from build123d import *

# Parameters (mm, degrees)
SKETCH_1_W                  = 84
SKETCH_1_H                  = 80
SKETCH_1_R                  = 14
EXTRUDE_1_DEPTH             = 5
EXTRUDE_2_DEPTH             = 22
CUT_EXTRUDE_3_REACH         = 79
HOLE_START                  = -42
HOLE_WIZARD_2_OUTLINE_R     = 1.7
HOLE_WIZARD_2_DEPTH         = 11
HOLE_WIZARD_2_2_OUTLINE_R   = 3
HOLE_WIZARD_2_2_OUTLINE_R_2 = 1.7
HOLE_WIZARD_2_2_DEPTH       = 3.4
HOLE_WIZARD_M4_2_D          = 3.3
SKETCH_14_R                 = 38
SKETCH_14_R_2               = 31.1
CUT_EXTRUDE_4_DEPTH         = 4
HOLE_WIZARD_3_D             = 3.2
HOLE_WIZARD_3_CBORE_D       = 6
HOLE_WIZARD_3_CBORE_DEPTH   = 3.4
CHAMFER_1_SIZE              = 23


# Read off the part's stored shape, not the designer's step: 打孔尺寸(%根据)内六角圆柱头螺钉的类型2
with BuildPart() as part:
    # 草图1 → 凸台-拉伸1 (new, symmetric)
    with BuildSketch(Plane.XY):
        Rectangle(SKETCH_1_W, SKETCH_1_H)
        Circle(SKETCH_1_R, mode=Mode.SUBTRACT)
    extrude(amount=EXTRUDE_1_DEPTH, both=True)

    # 草图6 → 凸台-拉伸2 (add)
    with BuildSketch(Plane.ZY.offset(42)):
        Polygon((-5, -14.766158372), (-5, -40), (-30, -40), (-33.816179908, -20.367456331), align=None)
    extrude_2 = extrude(amount=-EXTRUDE_2_DEPTH)

    # 切除-拉伸3: up to this plane
    cut_extrude_3_end = Plane(origin=(-42, -40, 5), z_dir=(0, 1, 0))
    # 草图7 → 切除-拉伸3 (cut, up to the surface)
    with BuildSketch(Plane(origin=(0, -13.292034521, 2.583709779), x_dir=(1, 0, 0), z_dir=(0, 0.9816271834476648, -0.19080899537654153)), mode=Mode.PRIVATE) as cut_extrude_3_sk1:
        with BuildLine():
            Line((-31, 37.081175318), (-29, 37.081175318))
            Line((-29, 37.081175318), (-29, 29.662905695))
            ThreePointArc((-29, 29.662905695), (-30, 13.725651762), (-31, 29.662905695))
            Line((-31, 29.662905695), (-31, 37.081175318))
        make_face()
    cut_extrude_3_tool1 = split(extrude(cut_extrude_3_sk1.sketch, amount=-CUT_EXTRUDE_3_REACH, mode=Mode.PRIVATE), bisect_by=cut_extrude_3_end, keep=Keep.BOTH, mode=Mode.PRIVATE)
    cut_extrude_3 = cut_extrude_3_tool1.solids().sort_by_distance((-30, -17.589666, -19.525688))[0]
    add(cut_extrude_3, mode=Mode.SUBTRACT)

    # 打孔尺寸(%根据)内六角圆柱头螺钉的类型2 outline → 打孔尺寸(%根据)内六角圆柱头螺钉的类型2 (cut)
    with BuildSketch(Plane.YZ.offset(HOLE_START)):
        with Locations((-35.310255285, -26.836727248)):
            Circle(HOLE_WIZARD_2_OUTLINE_R)
        with Locations((-24.512356267, -28.935626197)):
            Circle(HOLE_WIZARD_2_OUTLINE_R)
    hole_wizard_2 = extrude(amount=HOLE_WIZARD_2_DEPTH, mode=Mode.SUBTRACT)

    # Hole Wizard 2 2 outline → Hole Wizard 2 2 (cut)
    # profile 1 of 2: a face of its own
    with BuildSketch(Plane.YZ.offset(HOLE_START)):
        with Locations((-35.310255285, -26.836727248)):
            Circle(HOLE_WIZARD_2_2_OUTLINE_R)
        with Locations((-35.310255285, -26.836727248)):
            Circle(HOLE_WIZARD_2_2_OUTLINE_R_2, mode=Mode.SUBTRACT)
    # profile 2 of 2: a face of its own
    with BuildSketch(Plane.YZ.offset(HOLE_START)):
        with Locations((-24.512356267, -28.935626197)):
            Circle(HOLE_WIZARD_2_2_OUTLINE_R)
        with Locations((-24.512356267, -28.935626197)):
            Circle(HOLE_WIZARD_2_2_OUTLINE_R_2, mode=Mode.SUBTRACT)
    hole_wizard_2_2 = extrude(amount=HOLE_WIZARD_2_2_DEPTH, mode=Mode.SUBTRACT)

    # M4 螺纹孔2 (through all)
    with Locations(Plane(origin=(-20, 0, 0), x_dir=(0, 0, -1), z_dir=(1, 0, 0))):
        with Locations((28.935626197, -24.512356267), (26.836727248, -35.310255285)):
            hole_wizard_m4_2 = Hole(HOLE_WIZARD_M4_2_D / 2)

    # 草图14 → 切除-拉伸4 (cut)
    with BuildSketch(Plane.XY.offset(5)):
        Circle(SKETCH_14_R)
        Circle(SKETCH_14_R_2, mode=Mode.SUBTRACT)
    extrude(amount=-CUT_EXTRUDE_4_DEPTH, mode=Mode.SUBTRACT)

    # 镜向1: 凸台-拉伸2, 切除-拉伸3, 打孔尺寸(%根据)内六角圆柱头螺钉的类型2, Hole Wizard 2 2, M4 螺纹孔2 across plane
    add(extrude_2.mirror(Plane(origin=(0, 0, 0), x_dir=(0, 0, 1), z_dir=(1, 0, 0))))
    add(cut_extrude_3.mirror(Plane(origin=(0, 0, 0), x_dir=(0, 0, 1), z_dir=(1, 0, 0))), mode=Mode.SUBTRACT)
    add(hole_wizard_2.mirror(Plane(origin=(0, 0, 0), x_dir=(0, 0, 1), z_dir=(1, 0, 0))), mode=Mode.SUBTRACT)
    add(hole_wizard_2_2.mirror(Plane(origin=(0, 0, 0), x_dir=(0, 0, 1), z_dir=(1, 0, 0))), mode=Mode.SUBTRACT)
    add(hole_wizard_m4_2.mirror(Plane(origin=(0, 0, 0), x_dir=(0, 0, 1), z_dir=(1, 0, 0))), mode=Mode.SUBTRACT)

    # 打孔尺寸(%根据)内六角圆柱头螺钉的类型3 (through all)
    with Locations(Plane(origin=(0, 0, -5), x_dir=(-1, 0, 0), z_dir=(0, 0, -1))):
        with Locations((0, 34.5), (34.5, 0), (0, -34.5), (-34.5, 0)):
            CounterBoreHole(HOLE_WIZARD_3_D / 2, HOLE_WIZARD_3_CBORE_D / 2, HOLE_WIZARD_3_CBORE_DEPTH)

    # 倒角1
    chamfer_1_edges = [part.edges().sort_by_distance(p)[0] for p in [
        (42, 40, 0),
        (-42, 40, 0),
    ]]
    chamfer(chamfer_1_edges, length=CHAMFER_1_SIZE)


solid = part.part
CAD build for the part. Positions are in the model's coordinates, mm. A direction names the side the tool comes from. Round coordinates to 2 decimals unless told otherwise and drop trailing zeros. Loops run counter-clockwise (first coordinate to the right, second up) from the corner with the lowest first, then second, coordinate; pieces in that order, holes last. Notation, with made-up numbers: M -35.5,36 L 7.5,36 A25 cw 7.5,69 Z; hole C 0.25,-15 d7. An arc over 180 degrees is marked long. One line per question, with ' | ' between items. Start each with the question number.
Item 1: Cut at D-D, the plane y = 11.5. Write the cut outline in (x, z), plus the area to 3 significant figures.
Item 2: Two-plate mould, pull along Z, no slides. Class faces 1 (the flat face through (-6, -31, 1)), 2 (the flat face through (-36, -1, -1.6)), 3 (the cylindrical face through (-40.324, -32.449, -25.936)): pulls with the +Z half, pulls with the -Z half, needs draft (parallel to the pull), parting line crosses it, or undercut.
Item 3: Cut at C-C, the plane x = 34.5. Write the cut outline in (y, z), plus the area to 3 significant figures.
Item 4: Pin check, flat tips, straight feed: pin 1 Ø6.5 at (y, z) = (-36.5, -28) entering from -X; pin 2 Ø4.5 at (y, z) = (-35.31, -26.84) entering from +X; pin 3 Ø10 at (x, y) = (-13.5, 10) entering from -Z; pin 4 Ø5.5 at (x, y) = (-34.5, 0) entering from +Z. Stop position of each tip, or through.
Item 5: Wall check: line 1 (Y direction, x = 0, z = 4); line 2 (Y direction, x = -34, z = -27.5); line 3 (X direction, y = -16.5, z = -6). Give the ranges that are in metal, low to high.
Item 6: Cut at A-A, the plane x = 0. State how many separate pieces and enclosed holes the cut face has, plus the area to 3 significant figures.
Item 7: Which spindle directions (+Z, -Z, +X, -X, +Y, -Y) get a long thin tool onto all of the face, cutting with end or side? Do faces 4 (the flat face through (38.6, -25, -31)), 5 (the cylindrical face through (-40.324, -22.9, -26.406)), 6 (the flat face through (-3.3, -38.3, 5)), 7 (the cylindrical face through (-31.5, 0.1, -3.3)). Say none if no direction does.
Responses:
1) outline: M -42,-5 L -7.98,-5 L -7.98,5 L -28.9,5 L -28.9,1 L -36.22,1 L -36.22,5 L -42,5 Z; M 7.98,-5 L 42,-5 L 42,5 L 36.22,5 L 36.22,1 L 28.9,1 L 28.9,5 L 7.98,5 Z | area: 622 mm²
2) face 1: pulls with the +Z half | face 2: pulls with the -Z half | face 3: undercut
3) outline: M -40,-30 L -20.37,-33.82 L -18.7,-25.24 L -40,-21.1 Z; M -40,-7.62 L -16.18,-12.25 L -14.77,-5 L -3,-5 L -3,-1.6 L -1.6,-1.6 L -1.6,1 L -15.93,1 L -15.93,5 L -40,5 Z; M 1.6,-1.6 L 3,-1.6 L 3,-5 L 24.5,-5 L 24.5,5 L 15.93,5 L 15.93,1 L 1.6,1 Z; hole C -35.31,-26.84 d3.4; hole C -24.51,-28.94 d3.4 | area: 776 mm²
4) pin 1: stops at x = -42 | pin 2: stops at x = 38.6 | pin 3: stops at z = -5 | pin 4: stops at z = 1
5) line 1: y = -40 to -38, -31.1 to -14, 14 to 31.1, 38 to 40 | line 2: y = -40 to -36.88, -33.74 to -25.42, -23.6 to -19.14 | line 3: x = -42 to -20, 20 to 42
6) separate pieces: 4 | enclosed holes: 0 | area: 407 mm²
7) face 4: +X | face 5: -X | face 6: +Z, +X, -X, +Y, -Y | face 7: -Z
